Here's how the part is built. I have some questions about the finished solid (model axes, mm). A direction names the side the tool comes from. Coordinates: 2 decimals unless noted, no trailing zeros. Loops run counter-clockwise (first coordinate to the right, second up) from the corner with the lowest first, then second, coordinate; pieces in that order, holes last. Notation, with made-up numbers: (26.5, 21.25) -> (67.5, 21.25) arc R21 ccw to (67.5, 51.25) -> close; hole circle Ø2 at (59.25, -36.5). An arc over 180 degrees is marked (long way). Answer as a JSON object with one key per item and string values. Group by question number.
Q1. On a 3-axis mill with a long thin cutter (end or side, diameter ignored), from which of +Z, -Z, +X, -X, +Y, -Y can I reach the whole of each face in a straight line? I mean faces 3 (the flat face through (-4.1, 77.3, -77.5)), 4 (the flat face through (11.2, -0.4, -59.5)), 5 (the cylindrical face through (42.84, 15.793, -39.786)). Say none if no direction works.
Q2. I want a section at B-B on z = -31. Write out the boundary of the cut face in (x, y).
Q3. I'm going to push flat-ended pins straight in: pin 1 (6 mm diameter, centred on y = 8, z = -49.5, fed in from -X); pin 2 (0.8 mm diameter, centred on x = 2, y = 0.5, fed in from -Z); pin 3 (10 mm diameter, centred on y = 25.5, z = -53, fed in from +X). Where does each tip first touch, or does it pass through?
Q4. I need wall thicknesses on line 1 (X direction, y = 39, z = -28); line 2 (Y direction, x = 10, z = -58.5); line 3 (Z direction, x = -16, y = 50.5). Which ranges of each line are inside material? Lowest first, please.
Q5. I want a section at A-A on z = -68. Write out the boundary of the cut face in (x, y), then the cut area to 3 significant figures.
Q6. Thinking about a two-plate mould opening in Y: for faces 1 (the flat face through (11, 41, 0)), 2 (the flat face through (11, 41, 1.5)), which applies, released by +Y, released by -Y, zero draft, split by the parting line, or undercut?
```python
from build123d import *

# Parameters (mm, degrees)
ESQUISSE1_R             = 41.5
BOSS_EXTRU_1_DEPTH      = 1.5
BOSS_EXTRU_2_START      = 77.5
ESQUISSE2_R             = 41.5
ESQUISSE2_R_2           = 40
BOSS_EXTRU_2_DEPTH      = 77.5
ENL_V_MAT_EXTRU_2_DEPTH = 3
ENL_V_MAT_EXTRU_3_DEPTH = 15
FILLET1_R               = 1


with BuildPart() as part:
    # Esquisse1 → Boss.-Extru.1 (new body)
    with BuildSketch(Plane.XY):
        with Locations((11.097015348, 40.132293596)):
            Circle(ESQUISSE1_R)
    extrude(amount=BOSS_EXTRU_1_DEPTH)

    # Esquisse2 → Boss.-Extru.2 (add)
    with BuildSketch(Plane(origin=(0, 0, 0), x_dir=(-1, 0, 0), z_dir=(0, 0, -1)).offset(BOSS_EXTRU_2_START)):
        with Locations((-11.097015348, 40.132293596)):
            Circle(ESQUISSE2_R)
        with Locations((-11.097015348, 40.132293596)):
            Circle(ESQUISSE2_R_2, mode=Mode.SUBTRACT)
    extrude(amount=-BOSS_EXTRU_2_DEPTH)

    # Esquisse4 → Enlèv. mat.-Extru.2 (cut)
    with BuildSketch(Plane(origin=(0, 0, -77.5), x_dir=(-1, 0, 0), z_dir=(0, 0, -1))):
        with BuildLine():
            Line((-21.096949989, -0.144887377), (-21.096949989, 1.402443259))
            ThreePointArc((-21.096949989, 1.402443259), (-20.410817154, 1.231739668), (-19.721774233, 1.073190507))
            ThreePointArc((-19.721774233, 1.073190507), (-11.224690221, 0.132497358), (-2.721774233, 1.018928409))
            ThreePointArc((-2.721774233, 1.018928409), (-1.907360872, 1.202224875), (-1.096949989, 1.40247701))
            Line((-1.096949989, 1.40247701), (-1.096949989, -0.144854923))
            ThreePointArc((-1.096949989, -0.144854923), (-1.907510299, -0.337485214), (-2.721774233, -0.513805064))
            ThreePointArc((-2.721774233, -0.513805064), (-11.224476459, -1.367510664), (-19.721774233, -0.461591832))
            ThreePointArc((-19.721774233, -0.461591832), (-20.410708368, -0.309085242), (-21.096949989, -0.144887377))
        make_face()
    extrude(amount=-ENL_V_MAT_EXTRU_2_DEPTH, mode=Mode.SUBTRACT)

    # Esquisse5 → Enlèv. mat.-Extru.3 (cut)
    with BuildSketch(Plane(origin=(0, 0, -74.5), x_dir=(-1, 0, 0), z_dir=(0, 0, -1))):
        with BuildLine():
            Line((-19.597015348, 1.045850934), (-19.597015348, -0.487898427))
            ThreePointArc((-19.597015348, -0.487898427), (-11.097015348, -1.367706404), (-2.597015348, -0.487898427))
            Line((-2.597015348, -0.487898427), (-2.597015348, 1.045850934))
            ThreePointArc((-2.597015348, 1.045850934), (-11.097015348, 0.132293596), (-19.597015348, 1.045850934))
        make_face()
    extrude(amount=-ENL_V_MAT_EXTRU_3_DEPTH, mode=Mode.SUBTRACT)

    # Fillet1
    fillet1_edges = [part.edges().sort_by_distance(p)[0] for p in [
        (-30.402984652, 40.132293596, 1.5),
        (51.097015348, 40.132293596, 0),
    ]]
    fillet(fillet1_edges, radius=FILLET1_R)


solid = part.part
```
Result set:
{
 "1": {"face 3": "-Z, +X, -X, +Y, -Y", "face 4": "-Z, -Y", "face 5": "-Z"},
 "2": {"outline": "circle Ø83 at (11.1, 40.13); hole circle Ø80 at (11.1, 40.13)"},
 "3": {"pin 1": "stops at x = -18.46", "pin 2": "stops at z = -74.5", "pin 3": "stops at x = 51.46"},
 "4": {"line 1": "x = -30.39 to -28.89, 51.08 to 52.58", "line 2": "y = -1.35 to 0.15, 80.12 to 81.62", "line 3": "z = 0 to 1.5"},
 "5": {"outline": "(2.6, -0.49) -> (2.6, 1.05) arc R40 cw (long way) to (19.6, 1.05) -> (19.6, -0.49) arc R41.5 ccw (long way) to start", "area": "358 mm²"},
 "6": {"face 1": "undercut", "face 2": "zero draft"}
}
